Check sheet for the modelled part. Datum: model origin and axes. Units: mm. A direction names the side the tool comes from. Round coordinates to 2 decimals unless told otherwise and drop trailing zeros. Order: outer loops, then holes, each group sorted by start corner. A loop starts at its lowest first (then second) coordinate and runs counter-clockwise, first axis right, second up.
```python
from build123d import *

# Parameters (mm, degrees)
F0_R     = 4.5
F1_DEPTH = 8
F2_SIZE  = 3
F3_R     = 5
F4_R     = 1
F5_R     = 3


with BuildPart() as f1:
    # F0 (on Top) → F1 (new body)
    with BuildSketch(Plane.XY):
        with BuildLine():
            ThreePointArc((0, -12.5), (8.8388347648, -8.8388347648), (12.5, 0))
            ThreePointArc((12.5, 0), (8.8388347648, 8.8388347648), (0, 12.5))
            ThreePointArc((0, 12.5), (-12.5, 0), (0, -12.5))
        make_face()
        Circle(F0_R, mode=Mode.SUBTRACT)
        with BuildLine():
            ThreePointArc((0, -12.5), (-12.5, 0), (0, 12.5))
            Line((0, 12.5), (-52, 12.5))
            ThreePointArc((-52, 12.5), (-57.6568542495, 10.1568542495), (-60, 4.5))
            Line((-60, 4.5), (-60, -12.5))
            Line((-60, -12.5), (-53, -12.5))
            Line((-53, -12.5), (-53, 2.5))
            ThreePointArc((-53, 2.5), (-48, 4.7966687366), (-43, 2.5))
            Line((-43, 2.5), (-43, -12.5))
            Line((-43, -12.5), (0, -12.5))
        make_face()
    extrude(amount=F1_DEPTH)

    # F2
    f2_edges = [f1.edges().sort_by_distance(p)[0] for p in [
        (-43, -12.5, 4),
    ]]
    chamfer(f2_edges, length=F2_SIZE)

    # F3
    f3_edges = [f1.edges().sort_by_distance(p)[0] for p in [
        (-43, -9.5, 4),
    ]]
    fillet(f3_edges, radius=F3_R)

    # F4
    f4_edges = [f1.edges().sort_by_distance(p)[0] for p in [
        (-40, -12.5, 4),
    ]]
    fillet(f4_edges, radius=F4_R)

    # F5
    f5_edges = [f1.edges().sort_by_distance(p)[0] for p in [
        (-60, -12.5, 4),
    ]]
    fillet(f5_edges, radius=F5_R)


solid = f1.part
```
Item 1: Go/stop test with flat-tipped pins: P1, Ø1, axis at x = 4.5, z = 1, coming from the +Y side; P2, Ø2.5, axis at y = -5.5, z = 5.5, coming from the +X side. Record where each tip stops, or that it passes through.
Answer:
P1: stops at y = 11.84
P2: stops at x = 11.76
Item 2: Sectioned sample at A-A (z = 1). Record the cut outline in (x, y), and give its area (3 significant figures).
Answer:
outline: (-60, -9.5) arc R3 ccw to (-57, -12.5) - (-53, -12.5) - (-53, 2.5) arc R6.59 cw to (-43, 2.5) - (-43, -7.43) arc R5 ccw to (-41.54, -10.96) - (-40.29, -12.21) arc R1 ccw to (-39.59, -12.5) - (0, -12.5) arc R12.5 ccw to (0, 12.5) - (-52, 12.5) arc R8 ccw to (-60, 4.5) - close; hole circle Ø9 at (0, 0)
area: 1,500 mm2
Item 3: Sectioned sample at B-B (x = 8). Record the cut outline in (y, z), and give its area (3 significant figures).
Answer:
outline: (-9.6, 0) - (9.6, 0) - (9.6, 8) - (-9.6, 8) - close
area: 154 mm2
Item 4: Access from +Z, -Z, +X, -X, +Y, -Y to the whole of each face (thin tool, end or side, straight path). Record for faces 1 (the flat face through (-43, -2, 4)), 2 (the flat face through (-24, 0, 8)).
Answer:
face 1: +Z, -Z, -Y
face 2: +Z, +X, -X, +Y, -Y
Item 5: Sectioned sample at C-C (y = 5.5). Record the cut outline in (x, z), and give its area (3 significant figures).
Answer:
outline: (-59.94, 0) - (11.22, 0) - (11.22, 8) - (-59.94, 8) - close
area: 569 mm2
Item 6: Scan lines: line 1 along Y through (x, z) = (0, 5.5); line 2 along X through (y, z) = (-2, 2); line 3 along Y through (x, z) = (-45, 1.75). Record each from-to range of solid material in increasing order.
Answer:
line 1: y = -12.5 to -4.5, 4.5 to 12.5
line 2: x = -60 to -53, -43 to -4.03, 4.03 to 12.34
line 3: y = 4.07 to 12.5
Item 7: Release check for a two-part mould opening along X. For faces 3 (the flat face through (-26, 12.5, 4)), 4 (the flat face through (-40.9, -11.6, 3.9)), 5 (the flat face through (-60, -2, 4)) record: released by +X, released by -X, zero draft, split by the parting line, or undercut.
Answer:
face 3: zero draft
face 4: undercut
face 5: released by -X
